The figure shows three views and two pictorial views of one solid part (mm, origin at its lowest corner). Answer the questions. Round coordinates to 2 decimals unless told otherwise and drop trailing zeros. Loops run counter-clockwise (first coordinate to the right, second up) from the corner with the lowest first, then second, coordinate; pieces in that order, holes last. Notation, with made-up numbers: (51, 48.25) - (97, 48.25) arc R26 ccw to (97, 64.25) - close; hole circle Ø2 at (-7.75, -28). An arc over 180 degrees is marked (long way). Use one line per item in the form item = value. Start each with the question number.
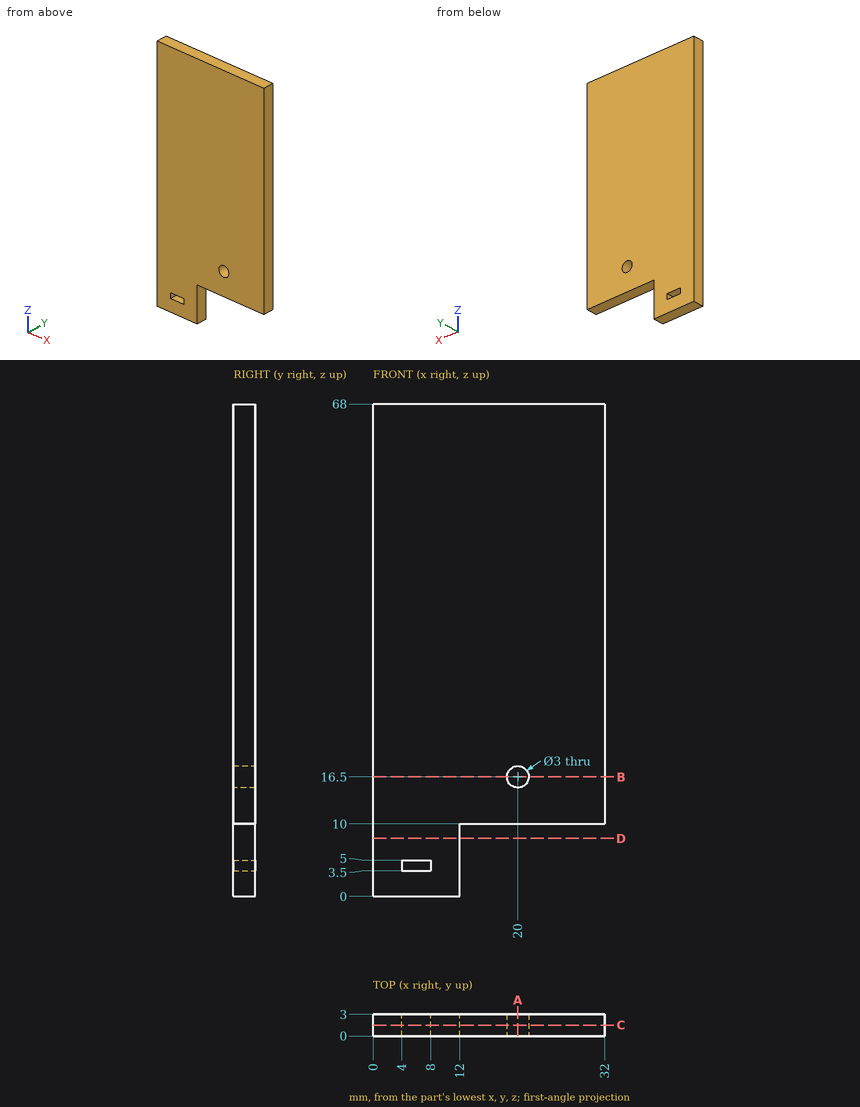
1) A cutting plane is placed at B-B on z = 16.5. Write down the section's boundary in (x, y), plus the area to 3 significant figures.
2) Straight lines are drawn through the part: line 1 (X direction, y = 1.5, z = 16.5); line 2 (Z direction, x = 17, y = 1.5); line 3 (Z direction, x = 21, y = 2.7). For each, find the intervals that lie inside material, in ascending order. Write a range as from..to.
3) A cutting plane is placed at A-A on x = 20. Write down the section's boundary in (y, z).
4) Flat-ended cylindrical pins translate along their axes: pin 1 (0.9 mm diameter, centred on y = 1.5, z = 7.5, fed in from +X); pin 2 (0.9 mm diameter, centred on x = 18, y = 1.5, fed in from -Z). Find the tip coordinate at first contact, or state that the pin passes through.
5) A cutting plane is placed at C-C on y = 1.5. Write down the section's boundary in (x, z).
6) A cutting plane is placed at D-D on z = 8. Write down the section's boundary in (x, y), plus the area to 3 significant figures.
Checks:
q1.outline = (0, 0) - (18.5, 0) - (18.5, 3) - (0, 3) - close; (21.5, 0) - (32, 0) - (32, 3) - (21.5, 3) - close
q1.area = 87.0 mm²
q2.line_1 = 0..18.5, 21.5..32
q2.line_2 = 10..68
q2.line_3 = 10..15.38, 17.62..68
q3.outline = (0, 10) - (3, 10) - (3, 15) - (0, 15) - close; (0, 18) - (3, 18) - (3, 68) - (0, 68) - close
q4.pin_1 = 12
q4.pin_2 = 10
q5.outline = (0, 0) - (12, 0) - (12, 10) - (32, 10) - (32, 68) - (0, 68) - close; hole (4, 3.5) - (8, 3.5) - (8, 5) - (4, 5) - close; hole circle Ø3 at (20, 16.5)
q6.outline = (0, 0) - (12, 0) - (12, 3) - (0, 3) - close
q6.area = 36.0 mm²
